Can you work these out from the model? Positions are in its coordinate system, mm. Give positions to 0.01 mm unless a question says otherwise; leave off trailing zeros. Order: outer loops, then holes, each group sorted by start corner. A loop starts at its lowest first (then second) coordinate and runs counter-clockwise, first axis right, second up. Notation, with made-up numbers: M 65,-23.5 L 118,-23.5 A34 cw 118,15.5 Z; hole C -21.5,77 d2. An arc over 180 degrees is marked long. Write each question's results on one line, items separated by ' | '.
from build123d import *

# Parameters (mm, degrees)
SKETCH1_W           = 101.6
SKETCH1_H           = 127
BOSS_EXTRUDE1_DEPTH = 6.35
SKETCH3_W           = 63.5
SKETCH3_H           = 127
SKETCH3_R           = 3.429
BOSS_EXTRUDE2_DEPTH = 6.35
SKETCH4_W           = 44.45
SKETCH4_H           = 127
CUT_EXTRUDE2_DEPTH  = 131.908603613
SKETCH5_R           = 2.54
CUT_EXTRUDE4_DEPTH  = 95.612869104


with BuildPart() as part:
    # Sketch1 → Boss-Extrude1 (new body)
    with BuildSketch(Plane(origin=(0, 0, 0), x_dir=(1, 0, 0), z_dir=(0, 1, 0))):
        Rectangle(SKETCH1_W, SKETCH1_H)
    extrude(amount=BOSS_EXTRUDE1_DEPTH)

    # Sketch3 → Boss-Extrude2 (add)
    with BuildSketch(Plane(origin=(0, 6.35, 0), x_dir=(1, 0, 0), z_dir=(0, 1, 0))):
        with Locations((-82.55, 0)):
            Rectangle(SKETCH3_W, SKETCH3_H)
        with Locations(Location((-101.6, 50.8, 0), (0, 0, 270))):
            Circle(SKETCH3_R, mode=Mode.SUBTRACT)
        with Locations(Location((-88.9, 50.8, 0), (0, 0, 270))):
            Circle(SKETCH3_R, mode=Mode.SUBTRACT)
        with Locations(Location((-88.9, 38.1, 0), (0, 0, 270))):
            Circle(SKETCH3_R, mode=Mode.SUBTRACT)
        with Locations(Location((-101.6, 38.1, 0), (0, 0, 270))):
            Circle(SKETCH3_R, mode=Mode.SUBTRACT)
        with Locations(Location((-101.6, 25.4, 0), (0, 0, 270))):
            Circle(SKETCH3_R, mode=Mode.SUBTRACT)
        with Locations(Location((-88.9, 25.4, 0), (0, 0, 270))):
            Circle(SKETCH3_R, mode=Mode.SUBTRACT)
        with Locations(Location((-76.2, 50.8, 0), (0, 0, 270))):
            Circle(SKETCH3_R, mode=Mode.SUBTRACT)
        with Locations(Location((-63.5, 50.8, 0), (0, 0, 270))):
            Circle(SKETCH3_R, mode=Mode.SUBTRACT)
        with Locations(Location((-76.2, 38.1, 0), (0, 0, 270))):
            Circle(SKETCH3_R, mode=Mode.SUBTRACT)
        with Locations(Location((-63.5, 38.1, 0), (0, 0, 270))):
            Circle(SKETCH3_R, mode=Mode.SUBTRACT)
        with Locations(Location((-76.2, 25.4, 0), (0, 0, 270))):
            Circle(SKETCH3_R, mode=Mode.SUBTRACT)
        with Locations(Location((-63.5, 25.4, 0), (0, 0, 270))):
            Circle(SKETCH3_R, mode=Mode.SUBTRACT)
        with Locations(Location((-101.6, 12.7, 0), (0, 0, 270))):
            Circle(SKETCH3_R, mode=Mode.SUBTRACT)
        with Locations(Location((-88.9, 12.7, 0), (0, 0, 270))):
            Circle(SKETCH3_R, mode=Mode.SUBTRACT)
        with Locations(Location((-76.2, 12.7, 0), (0, 0, 270))):
            Circle(SKETCH3_R, mode=Mode.SUBTRACT)
        with Locations(Location((-63.5, 12.7, 0), (0, 0, 270))):
            Circle(SKETCH3_R, mode=Mode.SUBTRACT)
        with Locations(Location((-101.6, 0, 0), (0, 0, 270))):
            Circle(SKETCH3_R, mode=Mode.SUBTRACT)
        with Locations(Location((-88.9, 0, 0), (0, 0, 270))):
            Circle(SKETCH3_R, mode=Mode.SUBTRACT)
        with Locations(Location((-76.2, 0, 0), (0, 0, 270))):
            Circle(SKETCH3_R, mode=Mode.SUBTRACT)
        with Locations(Location((-63.5, 0, 0), (0, 0, 270))):
            Circle(SKETCH3_R, mode=Mode.SUBTRACT)
        with Locations(Location((-101.6, -12.7, 0), (0, 0, 270))):
            Circle(SKETCH3_R, mode=Mode.SUBTRACT)
        with Locations(Location((-88.9, -12.7, 0), (0, 0, 270))):
            Circle(SKETCH3_R, mode=Mode.SUBTRACT)
        with Locations(Location((-76.2, -12.7, 0), (0, 0, 270))):
            Circle(SKETCH3_R, mode=Mode.SUBTRACT)
        with Locations(Location((-63.5, -12.7, 0), (0, 0, 270))):
            Circle(SKETCH3_R, mode=Mode.SUBTRACT)
        with Locations(Location((-101.6, -25.4, 0), (0, 0, 270))):
            Circle(SKETCH3_R, mode=Mode.SUBTRACT)
        with Locations(Location((-88.9, -25.4, 0), (0, 0, 270))):
            Circle(SKETCH3_R, mode=Mode.SUBTRACT)
        with Locations(Location((-76.2, -25.4, 0), (0, 0, 270))):
            Circle(SKETCH3_R, mode=Mode.SUBTRACT)
        with Locations(Location((-63.5, -25.4, 0), (0, 0, 270))):
            Circle(SKETCH3_R, mode=Mode.SUBTRACT)
        with Locations(Location((-101.6, -38.1, 0), (0, 0, 270))):
            Circle(SKETCH3_R, mode=Mode.SUBTRACT)
        with Locations(Location((-88.9, -38.1, 0), (0, 0, 270))):
            Circle(SKETCH3_R, mode=Mode.SUBTRACT)
        with Locations(Location((-76.2, -38.1, 0), (0, 0, 270))):
            Circle(SKETCH3_R, mode=Mode.SUBTRACT)
        with Locations(Location((-63.5, -38.1, 0), (0, 0, 270))):
            Circle(SKETCH3_R, mode=Mode.SUBTRACT)
        with Locations(Location((-101.6, -50.8, 0), (0, 0, 270))):
            Circle(SKETCH3_R, mode=Mode.SUBTRACT)
        with Locations(Location((-88.9, -50.8, 0), (0, 0, 270))):
            Circle(SKETCH3_R, mode=Mode.SUBTRACT)
        with Locations(Location((-76.2, -50.8, 0), (0, 0, 270))):
            Circle(SKETCH3_R, mode=Mode.SUBTRACT)
        with Locations(Location((-63.5, -50.8, 0), (0, 0, 270))):
            Circle(SKETCH3_R, mode=Mode.SUBTRACT)
    extrude(amount=-BOSS_EXTRUDE2_DEPTH)

    # Sketch4 → Cut-Extrude2 (cut, through all)
    with BuildSketch(Plane(origin=(0, 6.35, 0), x_dir=(1, 0, 0), z_dir=(0, 1, 0))):
        with Locations((-92.075, 0)):
            Rectangle(SKETCH4_W, SKETCH4_H)
    extrude(amount=-CUT_EXTRUDE2_DEPTH, mode=Mode.SUBTRACT)

    # Sketch5 → Cut-Extrude4 (cut, through all)
    with BuildSketch(Plane(origin=(0, 0, 0), x_dir=(1, 0, 0), z_dir=(0, 1, 0))):
        with Locations(Location((-50.8, 50.8, 0), (0, 0, 270))):
            Circle(SKETCH5_R)
        with Locations(Location((-50.8, 38.1, 0), (0, 0, 270))):
            Circle(SKETCH5_R)
        with Locations(Location((-50.8, 25.4, 0), (0, 0, 270))):
            Circle(SKETCH5_R)
        with Locations(Location((-50.8, 12.7, 0), (0, 0, 270))):
            Circle(SKETCH5_R)
        with Locations(Location((-50.8, 0, 0), (0, 0, 270))):
            Circle(SKETCH5_R)
        with Locations(Location((-50.8, -12.7, 0), (0, 0, 270))):
            Circle(SKETCH5_R)
        with Locations(Location((-50.8, -25.4, 0), (0, 0, 270))):
            Circle(SKETCH5_R)
        with Locations(Location((-50.8, -38.1, 0), (0, 0, 270))):
            Circle(SKETCH5_R)
        with Locations(Location((-50.8, -50.8, 0), (0, 0, 270))):
            Circle(SKETCH5_R)
    extrude(amount=CUT_EXTRUDE4_DEPTH, mode=Mode.SUBTRACT)


solid = part.part
(1) We'd pull the mould along Z, two halves only. Please class faces 1 (the face through (-48.66, 3.13, 52.17)), 2 (the face through (-10, 3, 63.5)), 3 (the face through (-10, 0, -1)), 4 (the face through (-65.59, 3.22, 22.68)): +Z half, -Z half, draft (parallel to the pull), parting line (faces both ways), or undercut.
Data:
face 1: undercut | face 2: +Z half | face 3: draft | face 4: undercut
(2) Imagine slicing it at B-B, the plane y = 1. Count the separate pieces of the cut face and the enclosed holes in it, plus the area to 3 significant figures.
Data:
separate pieces: 1 | enclosed holes: 18 | area: 14,800 mm2
(3) Imagine slicing it at D-D, the plane z = 24.5. Write out the boundary of the cut face in (x, y), plus the area to 3 significant figures.
Data:
outline: M -69.85,0 L -66.81,0 L -66.81,6.35 L -69.85,6.35 Z; M -60.19,0 L -53.18,0 L -53.18,6.35 L -60.19,6.35 Z; M -48.42,0 L 50.8,0 L 50.8,6.35 L -48.42,6.35 Z | area: 694 mm2
(4) Will these pins go through, and if not, where does the flat tip stop? P1, Ø4.5, axis at x = -50.8, z = 50.8, coming from the +Y side; P2, Ø5, axis at x = 17.5, z = 32.5, coming from the -Y side.
Data:
P1: passes through | P2: stops at y = 0
(5) Imagine slicing it at A-A, the plane z = -25.4. Write out the boundary of the cut face in (x, y).
Data:
outline: M -69.85,0 L -66.93,0 L -66.93,6.35 L -69.85,6.35 Z; M -60.07,0 L -53.34,0 L -53.34,6.35 L -60.07,6.35 Z; M -48.26,0 L 50.8,0 L 50.8,6.35 L -48.26,6.35 Z
(6) I need wall thicknesses on L1, parallel to X at y = 2, z = -12.7; L2, parallel to X at y = 4, z = 12; L3, parallel to X at y = 4, z = 28. Which ranges of each line are inside material? Lowest first, please. Write a range as from..to.
Data:
L1: x = -69.85..-66.93, -60.07..-53.34, -48.26..50.8 | L2: x = -69.85..-66.86, -60.14..-53.24, -48.36..50.8 | L3: x = -69.85..-65.74, -61.26..50.8
